Work out the finished part from the listing and answer in its coordinate system (mm). Coordinates: 2 decimals unless noted, no trailing zeros. Order: outer loops, then holes, each group sorted by start corner. A loop starts at its lowest first (then second) coordinate and runs counter-clockwise, first axis right, second up. Notation, with made-up numbers: M 53.25,3.25 L 75.25,3.25 A18 cw 75.25,19.25 Z; hole C 14.5,-35 d11. An arc over 180 degrees is marked long. Answer in a Markdown table with one row per item. Add a question column.
Item 1: A flat-ended cylindrical pin translates along its axis: pin 1 Ø2 at (y, z) = (9, 64) entering from +X. Find the tip coordinate at first contact, or state that the pin passes through.
Item 2: Consider line 1 (Y direction, x = -13, z = 12.5); line 2 (X direction, y = -2, z = 94); line 3 (X direction, y = 21, z = 15). Determine where each line is inside the solid, lowest interval first. Write a range as from..to.
Item 3: The part is cut by section A-A (y = 0). Write down the section's boundary in (x, z).
Item 4: The part is cut by section C-C (z = 65.5). State how many separate pieces and enclosed holes the cut face has, then the cut area to 3 significant figures.
Item 5: The part is cut by section B-B (x = -11). Write down the section's boundary in (y, z).
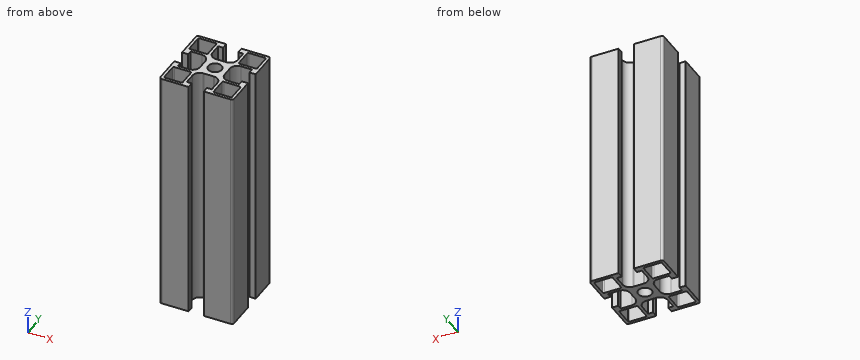
from build123d import *

# Parameters (mm, degrees)
SKETCH1_6_R         = 2.75
BOSS_EXTRUDE3_DEPTH = 100


with BuildPart() as part:
    # Sketch1_6 → Boss-Extrude3 (new body)
    with BuildSketch(Plane.XY):
        with BuildLine():
            Line((-8.207857566, 15.784975365), (-8.207857566, 13.784975365))
            Line((-8.207857566, 13.784975365), (-5.707857566, 13.784975365))
            Line((-5.707857566, 13.784975365), (-5.707857566, 24.684975365))
            ThreePointArc((-5.707857566, 24.684975365), (-6.000750784, 25.392082146), (-6.707857566, 25.684975365))
            Line((-6.707857566, 25.684975365), (-17.607857566, 25.684975365))
            Line((-17.607857566, 25.684975365), (-17.607857566, 23.184975365))
            Line((-17.607857566, 23.184975365), (-15.607857566, 23.184975365))
            Line((-15.607857566, 23.184975365), (-15.607857566, 18.878818393))
            Line((-15.607857566, 18.878818393), (-15.607857566, 18.684975365))
            ThreePointArc((-15.607857566, 18.684975365), (-16.432542315, 16.617397323), (-18.453822402, 15.684975365))
            ThreePointArc((-18.453822402, 15.684975365), (-18.61202607, 15.680806861), (-18.770229737, 15.684975365))
            Line((-18.770229737, 15.684975365), (-22.645485394, 15.684975365))
            ThreePointArc((-22.645485394, 15.684975365), (-22.803689062, 15.680806861), (-22.961892729, 15.684975365))
            ThreePointArc((-22.961892729, 15.684975365), (-24.983172816, 16.617397323), (-25.807857566, 18.684975365))
            Line((-25.807857566, 18.684975365), (-25.807857566, 18.878818393))
            Line((-25.807857566, 18.878818393), (-25.807857566, 23.184975365))
            Line((-25.807857566, 23.184975365), (-23.807857566, 23.184975365))
            Line((-23.807857566, 23.184975365), (-23.807857566, 25.684975365))
            Line((-23.807857566, 25.684975365), (-34.707857566, 25.684975365))
            ThreePointArc((-34.707857566, 25.684975365), (-35.414964347, 25.392082146), (-35.707857566, 24.684975365))
            Line((-35.707857566, 24.684975365), (-35.707857566, 13.784975365))
            Line((-35.707857566, 13.784975365), (-33.207857566, 13.784975365))
            Line((-33.207857566, 13.784975365), (-33.207857566, 15.784975365))
            Line((-33.207857566, 15.784975365), (-28.901700593, 15.784975365))
            Line((-28.901700593, 15.784975365), (-28.707857566, 15.784975365))
            ThreePointArc((-28.707857566, 15.784975365), (-26.640279523, 14.960290616), (-25.707857566, 12.939010529))
            ThreePointArc((-25.707857566, 12.939010529), (-25.703689062, 12.780806861), (-25.707857566, 12.622603193))
            Line((-25.707857566, 12.622603193), (-25.707857566, 8.747347537))
            ThreePointArc((-25.707857566, 8.747347537), (-25.703689062, 8.589143869), (-25.707857566, 8.430940201))
            ThreePointArc((-25.707857566, 8.430940201), (-26.640279523, 6.409660114), (-28.707857566, 5.584975365))
            Line((-28.707857566, 5.584975365), (-28.901700593, 5.584975365))
            Line((-28.901700593, 5.584975365), (-33.207857566, 5.584975365))
            Line((-33.207857566, 5.584975365), (-33.207857566, 7.584975365))
            Line((-33.207857566, 7.584975365), (-35.707857566, 7.584975365))
            Line((-35.707857566, 7.584975365), (-35.707857566, -3.315024635))
            ThreePointArc((-35.707857566, -3.315024635), (-35.414964347, -4.022131416), (-34.707857566, -4.315024635))
            Line((-34.707857566, -4.315024635), (-23.807857566, -4.315024635))
            Line((-23.807857566, -4.315024635), (-23.807857566, -1.815024635))
            Line((-23.807857566, -1.815024635), (-25.807857566, -1.815024635))
            Line((-25.807857566, -1.815024635), (-25.807857566, 2.491132338))
            Line((-25.807857566, 2.491132338), (-25.807857566, 2.684975365))
            ThreePointArc((-25.807857566, 2.684975365), (-24.983172816, 4.752553408), (-22.961892729, 5.684975365))
            ThreePointArc((-22.961892729, 5.684975365), (-22.803689062, 5.689143869), (-22.645485394, 5.684975365))
            Line((-22.645485394, 5.684975365), (-18.770229737, 5.684975365))
            ThreePointArc((-18.770229737, 5.684975365), (-18.61202607, 5.689143869), (-18.453822402, 5.684975365))
            ThreePointArc((-18.453822402, 5.684975365), (-16.432542315, 4.752553408), (-15.607857566, 2.684975365))
            Line((-15.607857566, 2.684975365), (-15.607857566, 2.491132338))
            Line((-15.607857566, 2.491132338), (-15.607857566, -1.815024635))
            Line((-15.607857566, -1.815024635), (-17.607857566, -1.815024635))
            Line((-17.607857566, -1.815024635), (-17.607857566, -4.315024635))
            Line((-17.607857566, -4.315024635), (-6.707857566, -4.315024635))
            ThreePointArc((-6.707857566, -4.315024635), (-6.000750784, -4.022131416), (-5.707857566, -3.315024635))
            Line((-5.707857566, -3.315024635), (-5.707857566, 7.584975365))
            Line((-5.707857566, 7.584975365), (-8.207857566, 7.584975365))
            Line((-8.207857566, 7.584975365), (-8.207857566, 5.584975365))
            Line((-8.207857566, 5.584975365), (-12.514014538, 5.584975365))
            Line((-12.514014538, 5.584975365), (-12.707857566, 5.584975365))
            ThreePointArc((-12.707857566, 5.584975365), (-14.775435608, 6.409660114), (-15.707857566, 8.430940201))
            ThreePointArc((-15.707857566, 8.430940201), (-15.71202607, 8.589143869), (-15.707857566, 8.747347537))
            Line((-15.707857566, 8.747347537), (-15.707857566, 12.622603193))
            ThreePointArc((-15.707857566, 12.622603193), (-15.71202607, 12.780806861), (-15.707857566, 12.939010529))
            ThreePointArc((-15.707857566, 12.939010529), (-14.775435608, 14.960290616), (-12.707857566, 15.784975365))
            Line((-12.707857566, 15.784975365), (-12.514014538, 15.784975365))
            Line((-12.514014538, 15.784975365), (-8.207857566, 15.784975365))
        make_face()
        with BuildLine():
            Line((-34.507857566, -2.63034887), (-34.507857566, 3.884975365))
            ThreePointArc((-34.507857566, 3.884975365), (-34.361410956, 4.238528756), (-34.007857566, 4.384975365))
            Line((-34.007857566, 4.384975365), (-27.507857566, 4.384975365))
            ThreePointArc((-27.507857566, 4.384975365), (-27.154304175, 4.238528756), (-27.007857566, 3.884975365))
            Line((-27.007857566, 3.884975365), (-27.007857566, -2.615024635))
            ThreePointArc((-27.007857566, -2.615024635), (-27.154304175, -2.968578025), (-27.507857566, -3.115024635))
            Line((-27.507857566, -3.115024635), (-34.023181801, -3.115024635))
            ThreePointArc((-34.023181801, -3.115024635), (-34.365899321, -2.97306639), (-34.507857566, -2.63034887))
        make_face(mode=Mode.SUBTRACT)
        with BuildLine():
            Line((-7.39253333, -3.115024635), (-13.907857566, -3.115024635))
            ThreePointArc((-13.907857566, -3.115024635), (-14.261410956, -2.968578025), (-14.407857566, -2.615024635))
            Line((-14.407857566, -2.615024635), (-14.407857566, 3.884975365))
            ThreePointArc((-14.407857566, 3.884975365), (-14.261410956, 4.238528756), (-13.907857566, 4.384975365))
            Line((-13.907857566, 4.384975365), (-7.407857566, 4.384975365))
            ThreePointArc((-7.407857566, 4.384975365), (-7.054304175, 4.238528756), (-6.907857566, 3.884975365))
            Line((-6.907857566, 3.884975365), (-6.907857566, -2.63034887))
            ThreePointArc((-6.907857566, -2.63034887), (-7.04981581, -2.97306639), (-7.39253333, -3.115024635))
        make_face(mode=Mode.SUBTRACT)
        with BuildLine():
            Line((-34.023181801, 24.484975365), (-27.507857566, 24.484975365))
            ThreePointArc((-27.507857566, 24.484975365), (-27.154304175, 24.338528756), (-27.007857566, 23.984975365))
            Line((-27.007857566, 23.984975365), (-27.007857566, 17.484975365))
            ThreePointArc((-27.007857566, 17.484975365), (-27.154304175, 17.131421975), (-27.507857566, 16.984975365))
            Line((-27.507857566, 16.984975365), (-34.007857566, 16.984975365))
            ThreePointArc((-34.007857566, 16.984975365), (-34.361410956, 17.131421975), (-34.507857566, 17.484975365))
            Line((-34.507857566, 17.484975365), (-34.507857566, 24.000299601))
            ThreePointArc((-34.507857566, 24.000299601), (-34.365899321, 24.34301712), (-34.023181801, 24.484975365))
        make_face(mode=Mode.SUBTRACT)
        with Locations((-20.707857566, 10.684975365)):
            Circle(SKETCH1_6_R, mode=Mode.SUBTRACT)
        with BuildLine():
            Line((-6.907857566, 24.000299601), (-6.907857566, 17.484975365))
            ThreePointArc((-6.907857566, 17.484975365), (-7.054304175, 17.131421975), (-7.407857566, 16.984975365))
            Line((-7.407857566, 16.984975365), (-13.907857566, 16.984975365))
            ThreePointArc((-13.907857566, 16.984975365), (-14.261410956, 17.131421975), (-14.407857566, 17.484975365))
            Line((-14.407857566, 17.484975365), (-14.407857566, 23.984975365))
            ThreePointArc((-14.407857566, 23.984975365), (-14.261410956, 24.338528756), (-13.907857566, 24.484975365))
            Line((-13.907857566, 24.484975365), (-7.39253333, 24.484975365))
            ThreePointArc((-7.39253333, 24.484975365), (-7.04981581, 24.34301712), (-6.907857566, 24.000299601))
        make_face(mode=Mode.SUBTRACT)
    extrude(amount=BOSS_EXTRUDE3_DEPTH)


solid = part.part
Reply:
| question | item | result |
|---|---|---|
| 1 | pin 1 | stops at x = -15.65 |
| 2 | line 1 | y = -4.32..-3.12, 4.38..5.6, 15.77..16.98, 24.48..25.68 |
| 2 | line 2 | x = -35.71..-34.51, -27.01..-23.81, -17.61..-14.41, -6.91..-5.71 |
| 2 | line 3 | x = -35.71..-34.51, -27.01..-25.81, -15.61..-14.41, -6.91..-5.71 |
| 3 | outline | M -35.71,0 L -34.51,0 L -34.51,100 L -35.71,100 Z; M -27.01,0 L -25.81,0 L -25.81,100 L -27.01,100 Z; M -15.61,0 L -14.41,0 L -14.41,100 L -15.61,100 Z; M -6.91,0 L -5.71,0 L -5.71,100 L -6.91,100 Z |
| 4 | separate pieces | 1 |
| 4 | enclosed holes | 5 |
| 4 | area | 299 mm2 |
| 5 | outline | M -4.32,0 L -3.12,0 L -3.12,100 L -4.32,100 Z; M 4.38,0 L 5.58,0 L 5.58,100 L 4.38,100 Z; M 15.78,0 L 16.98,0 L 16.98,100 L 15.78,100 Z; M 24.48,0 L 25.68,0 L 25.68,100 L 24.48,100 Z |
